```python
from build123d import *

# Parameters (mm, degrees)
F2_DEPTH  = 8.299
F4_DEPTH  = 3
F6_DEPTH  = 3
F8_DEPTH  = 8.299
F10_DEPTH = 3
F12_DEPTH = 8.299
F14_DEPTH = 3
F16_DEPTH = 8.299
F18_DEPTH = 3
F20_DEPTH = 10
F22_DEPTH = 10


with BuildPart() as f2:
    # F1 (on Top) → F2 (new body)
    with BuildSketch(Plane.XY):
        with BuildLine():
            ThreePointArc((-2.4485, 10), (-9.5195678119, 7.0710678119), (-12.4485, 0))
            Line((-12.4485, 0), (12.4485, 0))
            ThreePointArc((12.4485, 0), (9.5195678119, 7.0710678119), (2.4485, 10))
            Line((2.4485, 10), (0, 10))
            Line((0, 10), (-2.4485, 10))
        make_face()
    extrude(amount=F2_DEPTH)

    # F3 (on face) → F4 (join)
    with BuildSketch(Plane.XY.offset(8.299)):
        with BuildLine():
            ThreePointArc((17.4485, 0), (0, 17.4485), (-17.4485, 0))
            Line((-17.4485, 0), (17.4485, 0))
        make_face()
    extrude(amount=F4_DEPTH)

    # F5 (on face) → F6 (join)
    with BuildSketch(Plane(origin=(0, 0, 0), x_dir=(1, 0, 0), z_dir=(0, 0, -1))):
        with BuildLine():
            ThreePointArc((-25.7475, 0), (0, -25.7475), (25.7475, 0))
            Line((25.7475, 0), (-25.7475, 0))
        make_face()
    extrude(amount=F6_DEPTH)

    # F7 (on face) → F8 (join)
    with BuildSketch(Plane(origin=(0, 0, -3), x_dir=(1, 0, 0), z_dir=(0, 0, -1))):
        with BuildLine():
            ThreePointArc((7.7475, -13), (16.9398881554, -9.1923881554), (20.7475, 0))
            Line((20.7475, 0), (-20.7475, 0))
            ThreePointArc((-20.7475, 0), (-16.9398881554, -9.1923881554), (-7.7475, -13))
            Line((-7.7475, -13), (0, -13))
            Line((0, -13), (7.7475, -13))
        make_face()
    extrude(amount=F8_DEPTH)

    # F9 (on face) → F10 (join)
    with BuildSketch(Plane(origin=(0, 0, -11.299), x_dir=(1, 0, 0), z_dir=(0, 0, -1))):
        with BuildLine():
            ThreePointArc((-25.7475, 0), (0, -25.7475), (25.7475, 0))
            Line((25.7475, 0), (-25.7475, 0))
        make_face()
    extrude(amount=F10_DEPTH)

    # F11 (on face) → F12 (join)
    with BuildSketch(Plane(origin=(0, 0, -14.299), x_dir=(1, 0, 0), z_dir=(0, 0, -1))):
        with BuildLine():
            ThreePointArc((7.7475, -13), (16.9398881554, -9.1923881554), (20.7475, 0))
            Line((20.7475, 0), (-20.7475, 0))
            ThreePointArc((-20.7475, 0), (-16.9398881554, -9.1923881554), (-7.7475, -13))
            Line((-7.7475, -13), (0, -13))
            Line((0, -13), (7.7475, -13))
        make_face()
    extrude(amount=F12_DEPTH)

    # F13 (on face) → F14 (join)
    with BuildSketch(Plane(origin=(0, 0, -22.598), x_dir=(1, 0, 0), z_dir=(0, 0, -1))):
        with BuildLine():
            ThreePointArc((-25.7475, 0), (0, -25.7475), (25.7475, 0))
            Line((25.7475, 0), (-25.7475, 0))
        make_face()
    extrude(amount=F14_DEPTH)

    # F15 (on face) → F16 (join)
    with BuildSketch(Plane(origin=(0, 0, -25.598), x_dir=(1, 0, 0), z_dir=(0, 0, -1))):
        with BuildLine():
            Line((-2.4485, -10), (0, -10))
            Line((0, -10), (2.4485, -10))
            ThreePointArc((2.4485, -10), (9.5195678119, -7.0710678119), (12.4485, 0))
            Line((12.4485, 0), (0, 0))
            Line((0, 0), (-12.4485, 0))
            ThreePointArc((-12.4485, 0), (-9.5195678119, -7.0710678119), (-2.4485, -10))
        make_face()
    extrude(amount=F16_DEPTH)

    # F17 (on face) → F18 (join)
    with BuildSketch(Plane(origin=(0, 0, -33.897), x_dir=(1, 0, 0), z_dir=(0, 0, -1))):
        with BuildLine():
            ThreePointArc((-17.4485, 0), (0, -17.4485), (17.4485, 0))
            Line((17.4485, 0), (-17.4485, 0))
        make_face()
    extrude(amount=F18_DEPTH)

    # F19 (on face) → F20 (join)
    with BuildSketch(Plane.XZ):
        Polygon((0, -36.897), (17.4485, -36.897), (17.4485, -33.897), (12.4485, -33.897), (12.4485, -25.598), (25.7475, -25.598), (25.7475, -22.598), (20.7475, -22.598), (20.7475, -14.299), (25.7475, -14.299), (25.7475, -11.299), (20.7475, -11.299), (20.7475, -3), (25.7475, -3), (25.7475, 0), (12.4485, 0), (12.4485, 8.299), (17.4485, 8.299), (17.4485, 11.299), (0, 11.299), (-17.4485, 11.299), (-17.4485, 8.299), (-12.4485, 8.299), (-12.4485, 0), (-25.7475, 0), (-25.7475, -3), (-20.7475, -3), (-20.7475, -11.299), (-25.7475, -11.299), (-25.7475, -14.299), (-20.7475, -14.299), (-20.7475, -22.598), (-25.7475, -22.598), (-25.7475, -25.598), (-12.4485, -25.598), (-12.4485, -33.897), (-17.4485, -33.897), (-17.4485, -36.897), align=None)
    extrude(amount=F20_DEPTH)

    # F21 (on face) → F22 (cut)
    with BuildSketch(Plane.XZ.offset(10)):
        Polygon((-5.2, -36.897), (0, -36.897), (5.2, -36.897), (5.2, 11.299), (0, 11.299), (-5.2, 11.299), align=None)
    extrude(amount=-F22_DEPTH, mode=Mode.SUBTRACT)


solid = f2.part
```
Could you check a few things on this model? Use its own coordinates, in mm. A direction names the side the tool comes from. Coordinates: 2 decimals unless noted, no trailing zeros. Write each loop counter-clockwise with the first axis right and the second up, starting at its lowest first coordinate (ties: lowest second). Pieces come first, ordered by that corner, then holes. Notation, with made-up numbers: (43, -15.75) -> (57, -15.75) arc R24 ccw to (57, 17.25) -> close; hole circle Ø2 at (1, 28). An arc over 180 degrees is marked (long way). One line per question, with ' | ' between items. Start each with the question number.
1. Please list where these lines run through material, in increasing order: line 1 along Z through (x, y) = (3, 22); line 2 along Z through (x, y) = (15.5, -5.5); line 3 along X through (y, z) = (-7, -17).
2. Will these pins go through, and if not, where does the flat tip stop? P1, Ø8, axis at y = 7, z = -13, coming from the +X side; P2, Ø1.5, axis at x = 15, z = 0, coming from the +Y side; P3, Ø2.5, axis at x = -2.5, z = -18, coming from the +Y side.
3. Thinking about a two-plate mould opening in Z: for faces 1 (the face through (0, 4, -36.897)), 2 (the face through (-17.448, -5, -35)), 3 (the face through (0, 10, -30)), which applies, pulls with the +Z half, pulls with the -Z half, needs draft (parallel to the pull), parting line crosses it, or undercut?
4. If we section it at C-C (x = 21.5): Please give me the cut outline in (y, z).
5. If we section it at A-A (z = -32): Please give me the cut outline in (x, y).
6. If we section it at B-B (y = 15): Please give me the cut outline in (x, z).
7. For faces 4 (the face through (17.448, -5, 10)), 5 (the face through (0, 10, 4)), 6 (the face through (4.12, 10.02, -33.897)), 7 (the face through (-5.2, -5, -12)), 8 (the face through (17.448, -5, -35)), which set-ups out of +Z, -Z, +X, -X, +Y, -Y let a thin tool reach every point of the face, with its end or its side?
8. If we section it at D-D (x = 0): Please give me the cut outline in (y, z).
Return value:
1) line 1: z = -25.6 to -22.6, -14.3 to -11.3, -3 to 0 | line 2: z = -36.9 to -33.9, -25.6 to 0, 8.3 to 11.3 | line 3: x = -20.75 to -5.2, 5.2 to 20.75
2) P1: stops at x = 25.57 | P2: stops at y = 21.44 | P3: stops at y = 13
3) face 1: pulls with the -Z half | face 2: needs draft | face 3: undercut
4) outline: (-10, -25.6) -> (14.17, -25.6) -> (14.17, -22.6) -> (-10, -22.6) -> close; (-10, -14.3) -> (14.17, -14.3) -> (14.17, -11.3) -> (-10, -11.3) -> close; (-10, -3) -> (14.17, -3) -> (14.17, 0) -> (-10, 0) -> close
5) outline: (-12.45, -10) -> (-5.2, -10) -> (-5.2, 0) -> (5.2, 0) -> (5.2, -10) -> (12.45, -10) -> (12.45, 0) arc R10 ccw to (2.45, 10) -> (-2.45, 10) arc R10 ccw to (-12.45, 0) -> close
6) outline: (-20.93, -25.6) -> (20.93, -25.6) -> (20.93, -22.6) -> (-20.93, -22.6) -> close; (-20.93, -14.3) -> (20.93, -14.3) -> (20.93, -11.3) -> (-20.93, -11.3) -> close; (-20.93, -3) -> (20.93, -3) -> (20.93, 0) -> (-20.93, 0) -> close; (-8.91, -36.9) -> (8.91, -36.9) -> (8.91, -33.9) -> (-8.91, -33.9) -> close; (-8.91, 8.3) -> (8.91, 8.3) -> (8.91, 11.3) -> (-8.91, 11.3) -> close
7) face 4: +Z, +X, +Y, -Y | face 5: +X, -X, +Y | face 6: +Y | face 7: +Z, -Z, -Y | face 8: -Z, +X, +Y, -Y
8) outline: (0, -36.9) -> (17.45, -36.9) -> (17.45, -33.9) -> (10, -33.9) -> (10, -25.6) -> (25.75, -25.6) -> (25.75, -22.6) -> (13, -22.6) -> (13, -14.3) -> (25.75, -14.3) -> (25.75, -11.3) -> (13, -11.3) -> (13, -3) -> (25.75, -3) -> (25.75, 0) -> (10, 0) -> (10, 8.3) -> (17.45, 8.3) -> (17.45, 11.3) -> (0, 11.3) -> close
